Answer from the drawing. Dimensions are ordinates in mm from the lowest x, y and z of the part. A direction names the side the tool comes from. Coordinates: 2 decimals unless noted, no trailing zeros. Write each loop counter-clockwise with the first axis right and the second up, starting at its lowest first coordinate (ties: lowest second). Pieces come first, ordered by that corner, then holes.
(1) The mould has two halves that part along X. Classify the marked faces 1 and 2: +X half, -X half, draft (parallel to the pull), parting line (faces both ways), or undercut.
(2) Section A-A on x = 60.5 is taken. Write down the section's boundary in (y, z), then the cut area to 3 significant figures.
(3) Section C-C on y = 10 is taken. State how many separate pieces and enclosed holes the cut face has, then the cut area to 3 significant figures.
(4) Which of the six approach directions +Z, -Z, +X, -X, +Y, -Y give full straight-line access (tool end or side, diameter ignored) to the marked faces 3 and 4?
(5) Section D-D on x = 172.5 is taken. Write down the section's boundary in (y, z), then the cut area to 3 significant figures.
(6) Find the intervals of material crossed by probe 1 along Z at (x, y) = (77.5, 18.25); probe 2 along X at (y, z) = (7, 179) (1 decimal); probe 3 along X at (y, z) = (16.75, 57.5) (1 decimal), in increasing order.
(7) Section B-B on z = 212.5 is taken. Write down the section's boundary in (x, y) (1 decimal).
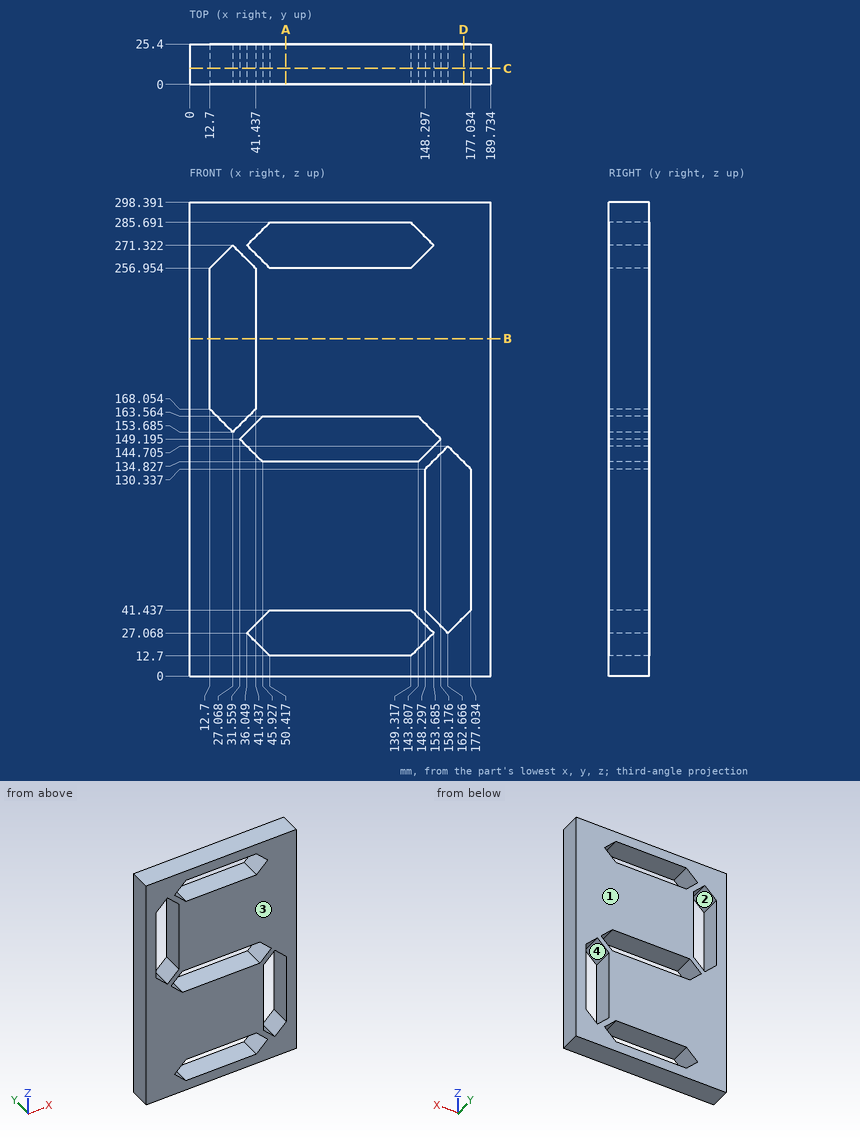
Response:
1. face 1: draft
1. face 2: undercut
2. outline: (0, 0) - (25.4, 0) - (25.4, 12.7) - (0, 12.7) - close; (0, 41.44) - (25.4, 41.44) - (25.4, 134.83) - (0, 134.83) - close; (0, 163.56) - (25.4, 163.56) - (25.4, 256.95) - (0, 256.95) - close; (0, 285.69) - (25.4, 285.69) - (25.4, 298.39) - (0, 298.39) - close
2. area: 5,390 mm2
3. separate pieces: 1
3. enclosed holes: 5
3. area: 41,500 mm2
4. face 3: +Z, -Z, +X, -X, -Y
4. face 4: +Y, -Y
5. outline: (0, 0) - (25.4, 0) - (25.4, 36.9) - (0, 36.9) - close; (0, 134.87) - (25.4, 134.87) - (25.4, 298.39) - (0, 298.39) - close
5. area: 5,090 mm2
6. probe 1: z = 0 to 12.7, 41.44 to 134.83, 163.56 to 256.95, 285.69 to 298.39
6. probe 2: x = 0 to 12.7, 41.4 to 189.7
6. probe 3: x = 0 to 148.3, 177 to 189.7
7. outline: (0, 0) - (12.7, 0) - (12.7, 25.4) - (0, 25.4) - close; (41.4, 0) - (189.7, 0) - (189.7, 25.4) - (41.4, 25.4) - close
